CAD build for the part. Positions are in the model's coordinates, mm. A direction names the side the tool comes from. Give positions to 0.01 mm unless a question says otherwise; leave off trailing zeros. Loops run counter-clockwise (first coordinate to the right, second up) from the corner with the lowest first, then second, coordinate; pieces in that order, holes last.
Item 1: Probe probe 1 along Y at (x, z) = (17, -6); probe 2 along X at (y, z) = (-47, 0); probe 3 along Y at (x, z) = (41.5, 5). List the from-to ranges inside material, lowest first.
Item 2: Saw through at D-D on x = 43. Give the cut face in (y, z) (1 decimal).
Item 3: Which spindle directions (+Z, -Z, +X, -X, +Y, -Y) get a long thin tool onto all of the face, cutting with end or side? Do faces 1 (the flat face through (0, -77.28, 0)), 2 (the flat face through (2.45, -6.22, 4.775)). Say none if no direction does.
Item 4: Mould opens along Y. For faces 3 (the cylindrical face through (29.24, -17.09, -0.13)), 4 (the flat face through (2, 71.946, 0)), 5 (the flat face through (75.756, -2, 0)) say: released by +Y, released by -Y, zero draft, split by the parting line, or undercut.
Item 5: Drop a flat-ended pin along its axis: P1, Ø21, axis at x = 0.5, y = 2, coming from the +Z side (3 decimals). Give the stop position or say it passes through.
Item 6: Saw through at A-A on y = 0. Give the cut face in (x, z) (1 decimal), plus the area to 3 significant figures.
Item 7: Saw through at C-C on z = 2. Give the number of separate pieces and of enclosed holes in the cut face, plus the area to 3 significant figures.
Item 8: Saw through at B-B on x = -0.5. Give the cut face in (y, z) (1 decimal), plus the area to 3 significant figures.
from build123d import *

# Parameters (mm, degrees)
F0_R           = 15.875
F1_DEPTH       = 9.525
F3_D           = 12.7
F3_CBORE_D     = 19.05
F3_CBORE_DEPTH = 4.7498


with BuildPart() as f1:
    # F0 (on Top) → F1 (new body, symmetric)
    with BuildSketch(Plane.XY):
        with BuildLine():
            Line((-67.1195, -77.2795), (69.4055, -77.2795))
            ThreePointArc((69.4055, -77.2795), (73.895628, -75.419628), (75.7555, -70.9295))
            Line((75.7555, -70.9295), (75.7555, 69.4055))
            ThreePointArc((75.7555, 69.4055), (75.011551, 71.201551), (73.2155, 71.9455))
            Line((73.2155, 71.9455), (-70.9295, 71.9455))
            ThreePointArc((-70.9295, 71.9455), (-72.725551, 71.201551), (-73.4695, 69.4055))
            Line((-73.4695, 69.4055), (-73.4695, -70.9295))
            ThreePointArc((-73.4695, -70.9295), (-71.609628, -75.419628), (-67.1195, -77.2795))
        make_face()
        with Locations((-29.0195, -32.8295)):
            Circle(F0_R, mode=Mode.SUBTRACT)
        with Locations((31.3055, -32.8295)):
            Circle(F0_R, mode=Mode.SUBTRACT)
        with Locations((-29.0195, 27.4955)):
            Circle(F0_R, mode=Mode.SUBTRACT)
        with Locations((31.3055, 27.4955)):
            Circle(F0_R, mode=Mode.SUBTRACT)
    extrude(amount=F1_DEPTH, both=True)

    # F3 (through all)
    with Locations(Plane.XY.offset(9.525)):
        with Locations((0.464717, 0)):
            CounterBoreHole(F3_D / 2, F3_CBORE_D / 2, F3_CBORE_DEPTH)


solid = f1.part
Results below:
1. probe 1: y = -77.28 to -39.71, -25.95 to 20.61, 34.38 to 71.95
1. probe 2: x = -73.47 to -36.18, -21.86 to 24.15, 38.46 to 75.76
1. probe 3: y = -77.28 to -45, -20.66 to 15.33, 39.66 to 71.95
2. outline: (-77.3, -9.5) - (-43.6, -9.5) - (-43.6, 9.5) - (-77.3, 9.5) - close; (-22.1, -9.5) - (16.8, -9.5) - (16.8, 9.5) - (-22.1, 9.5) - close; (38.2, -9.5) - (71.9, -9.5) - (71.9, 9.5) - (38.2, 9.5) - close
3. face 1: +Z, -Z, +X, -X, -Y
3. face 2: +Z
4. face 3: undercut
4. face 4: released by +Y
4. face 5: zero draft
5. P1: stops at z = 9.525
6. outline: (-73.5, -9.5) - (-5.9, -9.5) - (-5.9, 4.8) - (-9.1, 4.8) - (-9.1, 9.5) - (-73.5, 9.5) - close; (6.8, -9.5) - (75.8, -9.5) - (75.8, 9.5) - (10, 9.5) - (10, 4.8) - (6.8, 4.8) - close
6. area: 2,570 mm2
7. separate pieces: 1
7. enclosed holes: 5
7. area: 19,000 mm2
8. outline: (-77.3, -9.5) - (-6.3, -9.5) - (-6.3, 4.8) - (-9.5, 4.8) - (-9.5, 9.5) - (-77.3, 9.5) - close; (6.3, -9.5) - (71.9, -9.5) - (71.9, 9.5) - (9.5, 9.5) - (9.5, 4.8) - (6.3, 4.8) - close
8. area: 2,570 mm2
